Source: CAD feature listing. Evaluate the final solid. Frame: model axes, mm. A direction names the side the tool comes from. Give positions to 0.01 mm unless a question says otherwise; leave off trailing zeros. Loops run counter-clockwise (first coordinate to the right, second up) from the corner with the lowest first, then second, coordinate; pieces in that order, holes last.
from build123d import *

# Parameters (mm, degrees)
SKETCH1_R                = 100
BOSS_EXTRUDE1_DEPTH      = 5
CUT_EXTRUDE1_DEPTH       = 11
BOSS_EXTRUDE3_DEPTH      = 6
CHAMFER1_SIZE            = 1
CHAMFER2_SIZE            = 1
CHAMFER3_SIZE            = 1
CHAMFER1_OF_MIRROR1_SIZE = 1


with BuildPart() as part:
    # Sketch1 → Boss-Extrude1 (new body, symmetric)
    with BuildSketch(Plane.XY):
        Circle(SKETCH1_R)
    extrude(amount=BOSS_EXTRUDE1_DEPTH, both=True)

    # Sketch2 → Cut-Extrude1 (cut, through all)
    with BuildSketch(Plane.XY.offset(5)):
        with BuildLine():
            Line((6, 34.481879299), (6, 43.6))
            Line((6, 43.6), (-6, 43.6))
            Line((-6, 43.6), (-6, 34.481879299))
            ThreePointArc((-6, 34.481879299), (0, -35), (6, 34.481879299))
        make_face()
    extrude(amount=-CUT_EXTRUDE1_DEPTH, mode=Mode.SUBTRACT)

    # Sketch3 → Boss-Extrude3 (add)
    with BuildSketch(Plane.XY.offset(5)):
        with BuildLine():
            ThreePointArc((-7.489441028, 69.598191593), (0, 70), (7.489441028, 69.598191593))
            Line((7.489441028, 69.598191593), (9.629281322, 89.483389192))
            ThreePointArc((9.629281322, 89.483389192), (0, 90), (-9.629281322, 89.483389192))
            Line((-9.629281322, 89.483389192), (-7.489441028, 69.598191593))
        make_face()
        with BuildLine():
            ThreePointArc((-64.018522492, 28.313049606), (-60.621778265, 35), (-56.529081463, 41.285141987))
            Line((-56.529081463, 41.285141987), (-72.680247596, 53.080896841))
            ThreePointArc((-72.680247596, 53.080896841), (-77.942286341, 45), (-82.309528918, 36.402492351))
            Line((-82.309528918, 36.402492351), (-64.018522492, 28.313049606))
        make_face()
        with BuildLine():
            ThreePointArc((-56.529081463, -41.285141987), (-60.621778265, -35), (-64.018522492, -28.313049606))
            Line((-64.018522492, -28.313049606), (-82.309528918, -36.402492351))
            ThreePointArc((-82.309528918, -36.402492351), (-77.942286341, -45), (-72.680247596, -53.080896841))
            Line((-72.680247596, -53.080896841), (-56.529081463, -41.285141987))
        make_face()
        with BuildLine():
            ThreePointArc((7.489441028, -69.598191593), (0, -70), (-7.489441028, -69.598191593))
            Line((-7.489441028, -69.598191593), (-9.629281322, -89.483389192))
            ThreePointArc((-9.629281322, -89.483389192), (0, -90), (9.629281322, -89.483389192))
            Line((9.629281322, -89.483389192), (7.489441028, -69.598191593))
        make_face()
        with BuildLine():
            ThreePointArc((64.018522492, -28.313049606), (60.621778265, -35), (56.529081463, -41.285141987))
            Line((56.529081463, -41.285141987), (72.680247596, -53.080896841))
            ThreePointArc((72.680247596, -53.080896841), (77.942286341, -45), (82.309528918, -36.402492351))
            Line((82.309528918, -36.402492351), (64.018522492, -28.313049606))
        make_face()
        with BuildLine():
            ThreePointArc((56.529081463, 41.285141987), (60.621778265, 35), (64.018522492, 28.313049606))
            Line((64.018522492, 28.313049606), (82.309528918, 36.402492351))
            ThreePointArc((82.309528918, 36.402492351), (77.942286341, 45), (72.680247596, 53.080896841))
            Line((72.680247596, 53.080896841), (56.529081463, 41.285141987))
        make_face()
    boss_extrude3 = extrude(amount=BOSS_EXTRUDE3_DEPTH)

    # Chamfer1
    chamfer1_edges = [part.edges().sort_by_distance(p)[0] for p in [
        (0, 70, 11),
        (0, 90, 11),
        (-60.621778265, 35, 11),
        (-77.942286341, 45, 11),
        (-60.621778265, -35, 11),
        (-77.942286341, -45, 11),
        (0, -70, 11),
        (0, -90, 11),
        (60.621778265, -35, 11),
        (77.942286341, -45, 11),
        (60.621778265, 35, 11),
        (77.942286341, 45, 11),
    ]]
    chamfer(chamfer1_edges, length=CHAMFER1_SIZE)

    # Chamfer2
    chamfer2_edges = [part.edges().sort_by_distance(p)[0] for p in [
        (0, -35, -5),
        (0, -35, 5),
    ]]
    chamfer(chamfer2_edges, length=CHAMFER2_SIZE)

    # Chamfer3
    chamfer3_edges = [part.edges().sort_by_distance(p)[0] for p in [
        (-6, 43.6, 0),
        (6, 43.6, 0),
    ]]
    chamfer(chamfer3_edges, length=CHAMFER3_SIZE)

    # Mirror1: Boss-Extrude3 across plane
    add(boss_extrude3.mirror(Plane.XY))

    # Chamfer1 of Mirror1
    chamfer1_of_mirror1_edges = [part.edges().sort_by_distance(p)[0] for p in [
        (0, 70, -11),
        (0, 90, -11),
        (-60.621778265, 35, -11),
        (-77.942286341, 45, -11),
        (-60.621778265, -35, -11),
        (-77.942286341, -45, -11),
        (0, -70, -11),
        (0, -90, -11),
        (60.621778265, -35, -11),
        (77.942286341, -45, -11),
        (60.621778265, 35, -11),
        (77.942286341, 45, -11),
    ]]
    chamfer(chamfer1_of_mirror1_edges, length=CHAMFER1_OF_MIRROR1_SIZE)


solid = part.part
1) Cut plane A-A (y = 0). Return loops of the section in (x, z).
Checks:
outline: (-100, -5) - (-36, -5) - (-35, -4) - (-35, 4) - (-36, 5) - (-100, 5) - close; (35, -4) - (36, -5) - (100, -5) - (100, 5) - (36, 5) - (35, 4) - close
2) Contact query for flat-ended pins moving along their axis: P1, Ø12, axis at y = -67, z = 8, coming from the -X side; P2, Ø9, axis at y = 37.5, z = 0, coming from the +X side; P3, Ø1.5, axis at y = -20.5, z = -5.5, coming from the -X side; P4, Ø2, axis at x = -74.5, y = 32.5, coming from the -Z side. Output: stop coordinate, or through.
Checks:
P1: stops at x = -78.61
P2: stops at x = 94.4
P3: stops at x = -97.99
P4: stops at z = -11
3) Pull-direction query (X, two-part tool) for faces 4 (the flat face through (-8.574, 79.68, -7.958)), 5 (the cylindrical face through (78, 44.9, 7.5)), 6 (the flat face through (-64.718, -47.266, 7.958)); classes: released by +X, released by -X, zero draft, split by the parting line, or undercut.
Checks:
face 4: released by -X
face 5: released by +X
face 6: undercut
4) Cut plane C-C (z = -1.25). Return loops of the section in (x, y).
Checks:
outline: circle Ø200 at (0, 0); hole (-6, 34.48) arc R35 ccw (long way) to (6, 34.48) - (6, 42.6) - (5, 43.6) - (-5, 43.6) - (-6, 42.6) - close
5) Ray query, probe 1 along Z at (x, y) = (22, -63.5); probe 2 along Y at (x, z) = (-72, -10); probe 3 along Y at (x, z) = (-29.5, -1.5). Return the intervals inside material, ascending.
Checks:
probe 1: z = -5 to 5
probe 2: y = -52.58 to -31.84, 31.84 to 52.58
probe 3: y = -95.55 to -18.83, 18.83 to 95.55
6) Reachability of faces 1 (the cylindrical face through (0, 70, -7)), 2 (the flat face through (64.49, -47.1, 7.96)), 3 (the conical face through (-61.02, 35.11, 10.4)) from +Z, -Z, +X, -X, +Y, -Y: full face, straight path, thin tool, end or side. Return the list, or none.
Checks:
face 1: -Z
face 2: +Z, -Y
face 3: +Z
7) Cut plane D-D (x = -69). Return loops of the section in (y, z), and give its area (3 significant figures).
Checks:
outline: (-72.38, -5) - (-50.39, -5) - (-50.39, -11) - (-30.52, -11) - (-30.52, -5) - (30.52, -5) - (30.52, -11) - (50.39, -11) - (50.39, -5) - (72.38, -5) - (72.38, 5) - (50.39, 5) - (50.39, 11) - (30.52, 11) - (30.52, 5) - (-30.52, 5) - (-30.52, 11) - (-50.39, 11) - (-50.39, 5) - (-72.38, 5) - close
area: 1,920 mm2
